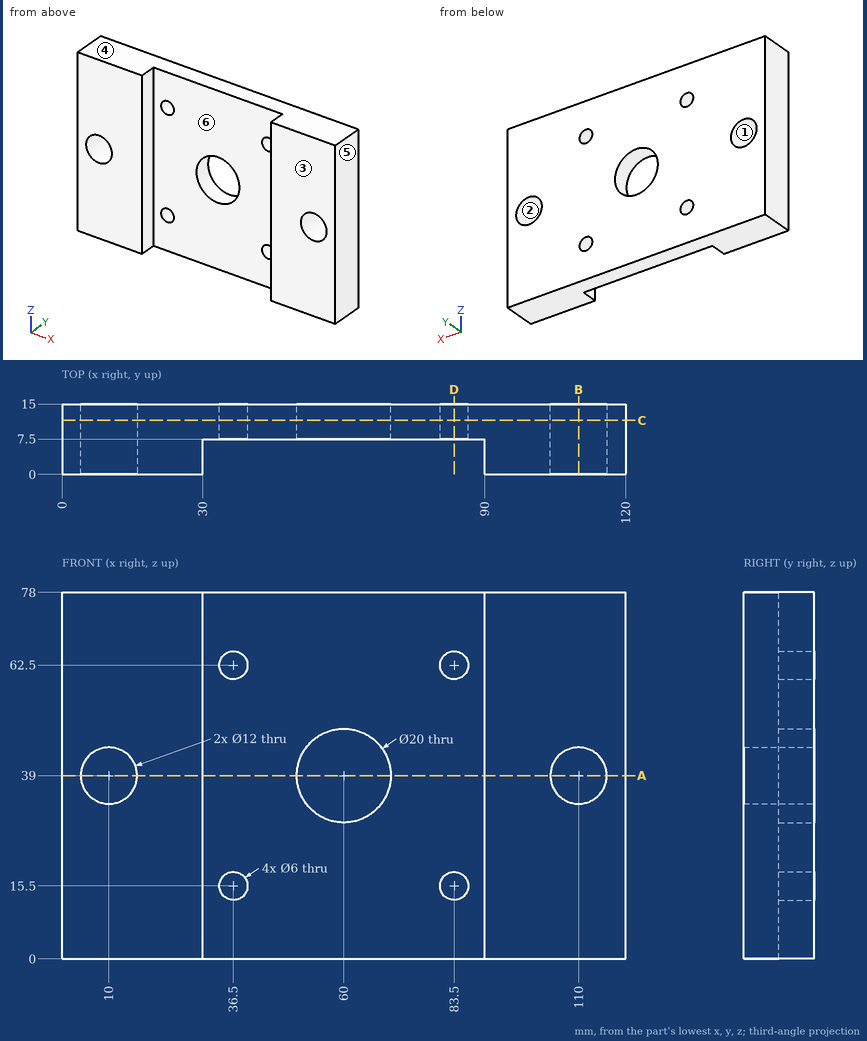
The drawing under review shows one solid part. Ordinate dimensions are in mm from its lowest x, y, z. A direction names the side the tool comes from. Give positions to 0.01 mm unless a question says otherwise; leave off trailing zeros. Order: outer loops, then holes, each group sorted by start corner. A loop starts at its lowest first (then second) coordinate and runs counter-clockwise, first axis right, second up. Notation, with made-up numbers: (-35, -27.5) -> (-30, -27.5) arc R22 cw to (-30, -9.5) -> close; hole circle Ø7 at (-32.75, 35.25). An arc over 180 degrees is marked (long way). Write item = value, one per line.
1) Draft analysis for pull direction Z (two halves, no side actions). For the marked faces 1, 2, 3 and 4, state which applies: pulls with the +Z half, pulls with the -Z half, needs draft (parallel to the pull), parting line crosses it, or undercut.
Findings:
face_1 = undercut
face_2 = undercut
face_3 = needs draft
face_4 = pulls with the +Z half
2) We need section B-B, the plane x = 110. Give the boundary of the cut face in (y, z), and give its area (3 significant figures).
Findings:
outline = (0, 0) -> (15, 0) -> (15, 33) -> (0, 33) -> close; (0, 45) -> (15, 45) -> (15, 78) -> (0, 78) -> close
area = 990 mm^2
3) Insertion check: pin 1 (10 mm diameter, centred on x = 65.5, z = 46.5, fed in from -Y). The pin has a flat end and moves straight along its axis. Give the tip position at first contact, or say it passes through.
Findings:
pin_1 = 7.5
4) We need section C-C, the plane y = 11.5. Give the boundary of the cut face in (x, z), and give its area (3 significant figures).
Findings:
outline = (0, 0) -> (120, 0) -> (120, 78) -> (0, 78) -> close; hole circle Ø12 at (10, 39); hole circle Ø6 at (36.5, 15.5); hole circle Ø6 at (36.5, 62.5); hole circle Ø20 at (60, 39); hole circle Ø6 at (83.5, 15.5); hole circle Ø6 at (83.5, 62.5); hole circle Ø12 at (110, 39)
area = 8,710 mm^2
5) We need section A-A, the plane z = 39. Give the boundary of the cut face in (x, y), and give its area (3 significant figures).
Findings:
outline = (0, 0) -> (4, 0) -> (4, 15) -> (0, 15) -> close; (16, 0) -> (30, 0) -> (30, 7.5) -> (50, 7.5) -> (50, 15) -> (16, 15) -> close; (70, 7.5) -> (90, 7.5) -> (90, 0) -> (104, 0) -> (104, 15) -> (70, 15) -> close; (116, 0) -> (120, 0) -> (120, 15) -> (116, 15) -> close
area = 840 mm^2
6) We need section D-D, the plane x = 83.5. Give the boundary of the cut face in (y, z).
Findings:
outline = (7.5, 0) -> (15, 0) -> (15, 12.5) -> (7.5, 12.5) -> close; (7.5, 18.5) -> (15, 18.5) -> (15, 59.5) -> (7.5, 59.5) -> close; (7.5, 65.5) -> (15, 65.5) -> (15, 78) -> (7.5, 78) -> close
7) For the marked faces 5 and 6, list the 3-axis set-ups (+Z, -Z, +X, -X, +Y, -Y) from which the entire face can be reached by the end or side of a thin tool; tool diameter is ignored.
Findings:
face_5 = +Z, -Z, +X, +Y, -Y
face_6 = +Z, -Z, -Y
8) To check wall thickness, follow L1, parallel to Z at x = 36.5, y = 12.75; L2, parallel to X at y = 4.75, z = 9; L3, parallel to X at y = 10.25, z = 40. State the ranges of each line that lie inside material, in increasing order. Write a range as from..to.
Findings:
L1 = 0..12.5, 18.5..59.5, 65.5..78
L2 = 0..30, 90..120
L3 = 0..4.08, 15.92..50.05, 69.95..104.08, 115.92..120
